```python
from build123d import *

# Parameters (mm, degrees)
FILLET1_R               = 1
CUT_EXTRUDE1_DEPTH      = 184.811724327
CUT_EXTRUDE1_DEPTH_BACK = 184.811724327
CUT_EXTRUDE2_DEPTH      = 183.746332303
CUT_EXTRUDE2_DEPTH_BACK = 180
SKETCH3_R               = 1.85
CUT_EXTRUDE3_DEPTH      = 184.811724344
CUT_EXTRUDE3_DEPTH_BACK = 184.811724344
SKETCH4_R               = 16


with BuildPart() as part:
    # Sketch1 → Revolve2 (revolve)
    with BuildSketch(Plane.XY, mode=Mode.PRIVATE) as revolve2_sk:
        Polygon((0, 0), (15.5, 0), (15.5, 46), (13.5, 75), (12.425, 75), (12.425, 157), (6.875, 157), (6.875, 179.1), (6.070935316, 179.1), (6.070935316, 180.55), (6.870935316, 180.55), (6.870935316, 182.5), (0, 182.5), align=None)
    revolve(revolve2_sk.sketch.rotate(Axis((0, 263.878189578, 0), (0, -1, 0)), 90), axis=Axis((0, 263.878189578, 0), (0, -1, 0)))

    # Fillet1
    fillet1_edges = [part.edges().sort_by_distance(p)[0] for p in [
        (0, 157, -12.425),
    ]]
    fillet(fillet1_edges, radius=FILLET1_R)

    # Sketch2 → Cut-Extrude1 (cut, two sides: drawn at the far end of the back side and taken through both)
    with BuildSketch(Plane.XY.offset(-CUT_EXTRUDE1_DEPTH_BACK)):
        with BuildLine():
            Line((-15.5, 3), (-19.676433944, 0))
            Line((-19.676433944, 0), (9.520360954, -11.635719705))
            Line((9.520360954, -11.635719705), (20.15271979, -0.609569802))
            Line((20.15271979, -0.609569802), (15.5, 12))
            add(Edge.make_bspline(
                [(15.5, 12), (5.345045333, -3.515489974), (-15.5, 3)],
                knots=[0, 0, 0, 1, 1, 1], degree=2))
        make_face()
    extrude(amount=CUT_EXTRUDE1_DEPTH + CUT_EXTRUDE1_DEPTH_BACK, mode=Mode.SUBTRACT)

    # Sketch3 → Cut-Extrude2 (cut, two sides: drawn at the far end of the back side and taken through both)
    with BuildSketch(Plane(origin=(0, 182.5, 0), x_dir=(1, 0, 0), z_dir=(0, 1, 0)).offset(-CUT_EXTRUDE2_DEPTH_BACK)):
        with Locations(Location((0, 0, 0), (0, 0, 90))):
            Circle(SKETCH3_R)
    extrude(amount=CUT_EXTRUDE2_DEPTH + CUT_EXTRUDE2_DEPTH_BACK, mode=Mode.SUBTRACT)

    # Sketch4 → Cut-Extrude3 (cut, two sides: drawn at the far end of the back side and taken through both)
    with BuildSketch(Plane(origin=(0, 0, 0), x_dir=(0, 0, -1), z_dir=(1, 0, 0)).offset(-CUT_EXTRUDE3_DEPTH_BACK)):
        with Locations((0, -5.093252724)):
            Circle(SKETCH4_R)
    extrude(amount=CUT_EXTRUDE3_DEPTH + CUT_EXTRUDE3_DEPTH_BACK, mode=Mode.SUBTRACT)


solid = part.part
```
Verification items for the finished model (mm, model axes). A direction names the side the tool comes from. Coordinates: 2 decimals unless noted, no trailing zeros. Write each loop counter-clockwise with the first axis right and the second up, starting at its lowest first coordinate (ties: lowest second). Pieces come first, ordered by that corner, then holes. Notation, with made-up numbers: M 75.25,37 L 85.25,37 A17 ccw 85.25,66 Z; hole C -11.5,84.5 d10. An arc over 180 degrees is marked long. Answer as a JSON object with one key per item and string values. Group by question number.
(1) Material ranges on line 1 (X direction, y = 57, z = 0); line 2 (X direction, y = 120, z = 0) (3 decimals); line 3 (Y direction, x = -8, z = 0.5), recorded low to high.
(2) Cross-section at A-A, the plane y = 154.5. Record the cut outline in (x, z) (3 decimals).
(3) Tool access check on faces 4 (the face through (5, 157, 5)), 5 (the face through (-6.02, 179.84, -0.79)), 6 (the face through (2.766, 10.905, -0.263)). Record the directions out of +Z, -Z, +X, -X, +Y, -Y that give a thin tool (end or side, any length) a straight path to the whole face; none if there is none.
(4) Gauge pin test, flat ends, axial feed: pin 1 (12 mm diameter, centred on x = 6.5, y = 160, fed in from +Z); pin 2 (2 mm diameter, centred on x = 11, y = 75, fed in from -Z); pin 3 (2 mm diameter, centred on y = 143, z = -1, fed in from +X) (3 decimals). Record the tip position at first contact, or that the pin passes through.
(5) Cross-section at B-B, the plane y = 73. Record the cut outline in (x, z), and give its area (3 significant figures).
(6) Release check for a two-part mould opening along X. For faces 1 (the face through (1.806, 95.446, 0.401)), 2 (the face through (1.43, 182.5, 1.43)), 3 (the face through (-13.07, 23.85, 8.33)) record: +X half, -X half, draft (parallel to the pull), parting line (faces both ways), or undercut.
Reply:
{
 "1": {"line 1": "-14.74 to -1.85, 1.85 to 14.74", "line 2": "-12.425 to -1.85, 1.85 to 12.425", "line 3": "10.9 to 157"},
 "2": {"outline": "C 0,0 d24.85; hole C 0,0 d3.7"},
 "3": {"face 4": "+Y", "face 5": "none", "face 6": "+X, -X, -Y"},
 "4": {"pin 1": "z = 12.27", "pin 2": "z = -9.07", "pin 3": "x = 12.425"},
 "5": {"outline": "C 0,0 d27.28; hole C 0,0 d3.7", "area": "574 mm²"},
 "6": {"face 1": "undercut", "face 2": "draft", "face 3": "parting line"}
}
